Geometry: final body of the model. Coordinates: model frame, mm. Give positions to 0.01 mm unless a question says otherwise; leave off trailing zeros. Loops run counter-clockwise (first coordinate to the right, second up) from the corner with the lowest first, then second, coordinate; pieces in that order, holes last. Notation, with made-up numbers: M 27.5,50.25 L 53.5,50.25 A19 cw 53.5,63.25 Z; hole C 22.5,-5.5 d8. An arc over 180 degrees is marked long. One line per question, with ' | ' between items. Start each with the question number.
from build123d import *

# Parameters (mm, degrees)
SKETCH1_W           = 20
SKETCH1_H           = 28
BOSS_EXTRUDE1_DEPTH = 1.5
BOSS_EXTRUDE2_DEPTH = 0.1
FILLET1_R           = 2


with BuildPart() as part:
    # Sketch1 → Boss-Extrude1 (new body)
    with BuildSketch(Plane(origin=(0, 0, 0), x_dir=(1, 0, 0), z_dir=(0, 1, 0))):
        with Locations((10, 14)):
            Rectangle(SKETCH1_W, SKETCH1_H)
    extrude(amount=BOSS_EXTRUDE1_DEPTH)

    # Sketch2 → Boss-Extrude2 (add)
    with BuildSketch(Plane(origin=(0, 1.5, 0), x_dir=(1, 0, 0), z_dir=(0, 1, 0))):
        with BuildLine():
            Line((5.5, 17), (14.5, 17))
            ThreePointArc((14.5, 17), (15.914213562, 16.414213562), (16.5, 15))
            Line((16.5, 15), (16.5, 6))
            ThreePointArc((16.5, 6), (15.914213562, 4.585786438), (14.5, 4))
            Line((14.5, 4), (5.5, 4))
            ThreePointArc((5.5, 4), (4.085786438, 4.585786438), (3.5, 6))
            Line((3.5, 6), (3.5, 15))
            ThreePointArc((3.5, 15), (4.085786438, 16.414213562), (5.5, 17))
        make_face()
    extrude(amount=BOSS_EXTRUDE2_DEPTH)

    # Fillet1
    fillet1_edges = [part.edges().sort_by_distance(p)[0] for p in [
        (0, 0.75, -28),
        (20, 0.75, -28),
        (20, 0.75, 0),
        (0, 0.75, 0),
    ]]
    fillet(fillet1_edges, radius=FILLET1_R)


solid = part.part
Q1. Section B-B, the plane x = 9.75. Output: boundary loops of the cut face in (y, z).
Q2. Material intervals for L1, parallel to Y at x = 14.25, z = -2; L2, parallel to Z at x = 18.75, y = 0.7; L3, parallel to X at y = 0.4, z = -1.5, sorted ascending.
Q3. Section A-A, the plane z = -12.5. Output: boundary loops of the cut face in (x, y).
Q4. Section C-C, the plane x = 18.5. Output: boundary loops of the cut face in (y, z).
Q5. Contact query for a flat-ended pin moving along its axis: pin 1 (4 mm diameter, centred on x = 3.5, z = -16, fed in from -Y). Output: stop coordinate, or through.
Model answer:
1) outline: M 0,-28 L 1.5,-28 L 1.5,-17 L 1.6,-17 L 1.6,-4 L 1.5,-4 L 1.5,0 L 0,0 Z
2) L1: y = 0 to 1.5 | L2: z = -27.85 to -0.15 | L3: x = 0.06 to 19.94
3) outline: M 0,0 L 20,0 L 20,1.5 L 16.5,1.5 L 16.5,1.6 L 3.5,1.6 L 3.5,1.5 L 0,1.5 Z
4) outline: M 0,-27.94 L 1.5,-27.94 L 1.5,-0.06 L 0,-0.06 Z
5) pin 1: stops at y = 0
